from build123d import *

# Parameters (mm, degrees)
BOSS_EXTRUDE1_DEPTH   = 10
FILLET1_R             = 2
F_3_0MM_DOWEL_HOLE1_D = 3.5
F_3_0MM_DOWEL_HOLE2_D = 3.5


with BuildPart() as part:
    # Sketch1 → Boss-Extrude1 (new body)
    with BuildSketch(Plane.XY):
        Polygon((0, 0), (14, 0), (14, 42), (25, 42), (25, 45), (11, 45), (11, 3), (0, 3), align=None)
    extrude(amount=-BOSS_EXTRUDE1_DEPTH)

    # Fillet1
    fillet1_edges = [part.edges().sort_by_distance(p)[0] for p in [
        (11, 3, -5),
        (11, 45, -5),
        (14, 42, -5),
        (14, 0, -5),
    ]]
    fillet(fillet1_edges, radius=FILLET1_R)

    # Ø3.0mm Dowel Hole1 (through all)
    with Locations(Plane(origin=(4.5, 0, -5), x_dir=(0, 0, -1), z_dir=(0, -1, 0))):
        with Locations((0, 0)):
            Hole(F_3_0MM_DOWEL_HOLE1_D / 2)

    # Ø3.0mm Dowel Hole2 (through all)
    with Locations(Plane(origin=(0, 45, 0), x_dir=(1, 0, 0), z_dir=(0, 1, 0))):
        with Locations((20.5, 5)):
            Hole(F_3_0MM_DOWEL_HOLE2_D / 2)


solid = part.part
The listing builds one solid part. Answer for the finished solid, in the listing's coordinates (mm). A direction names the side the tool comes from. Coordinates: 2 decimals unless noted, no trailing zeros. Loops run counter-clockwise (first coordinate to the right, second up) from the corner with the lowest first, then second, coordinate; pieces in that order, holes last. Notation, with made-up numbers: (61, 65.5) -> (78, 65.5) arc R24 cw to (78, 79.5) -> close; hole circle Ø7 at (77, -38). An arc over 180 degrees is marked (long way). Write item = value, one per line. Start each with the question number.
1) A cutting plane is placed at A-A (z = -5). Give the vertices of the cut face in (x, y), then the cut area to 3 significant figures.
2) The mould has two halves that part along X. Classify faces 4 (the face through (10.43, 3.6, -5.07)), 5 (the face through (21.89, 43.48, -3.94)), 6 (the face through (12, 23, -10)): released by +X, released by -X, zero draft, split by the parting line, or undercut.
3) A cutting plane is placed at C-C (z = -2.5). Give the vertices of the cut face in (x, y), then the cut area to 3 significant figures.
4) Straight lines are drawn through the part: line 1 (X direction, y = 42.8, z = -5); line 2 (Y direction, x = 2, z = -7); line 3 (X direction, y = 22.5, z = -6.75). For each, find the intervals that lie inside material, in ascending order. Write a range as from..to.
5) Given pin 1 Ø1.5 at (y, z) = (29, -4) entering from +X; pin 2 Ø5 at (x, z) = (17, -8) entering from -Y; pin 3 Ø1.5 at (y, z) = (40, -5) entering from +X, each flat-ended and moving along its own axis, determine where each tip first touches the part or whether it passes through.
6) A tool of negligible diameter and unlimited length cuts with its end or side. For faces 1 (the face through (0, 2, -5)), 2 (the face through (18, 42, -5)), 3 (the face through (11, 24, -5)), from which of +Z, -Z, +X, -X, +Y, -Y can it reach the whole face along a straight path? Write none if from no direction.
7) A cutting plane is placed at B-B (x = 20.5). Give the vertices of the cut face in (y, z), then the cut area to 3 significant figures.
8) A cutting plane is placed at D-D (y = 23). Give the vertices of the cut face in (x, z), then the cut area to 3 significant figures.
Responses:
q1.outline = (0, 0) -> (2.75, 0) -> (2.75, 3) -> (0, 3) -> close; (6.25, 0) -> (12, 0) arc R2 ccw to (14, 2) -> (14, 40) arc R2 cw to (16, 42) -> (18.75, 42) -> (18.75, 45) -> (13, 45) arc R2 ccw to (11, 43) -> (11, 5) arc R2 cw to (9, 3) -> (6.25, 3) -> close; (22.25, 42) -> (25, 42) -> (25, 45) -> (22.25, 45) -> close
q1.area = 180 mm²
q2.face_4 = released by -X
q2.face_5 = undercut
q2.face_6 = zero draft
q3.outline = (0, 0) -> (12, 0) arc R2 ccw to (14, 2) -> (14, 40) arc R2 cw to (16, 42) -> (25, 42) -> (25, 45) -> (13, 45) arc R2 ccw to (11, 43) -> (11, 5) arc R2 cw to (9, 3) -> (0, 3) -> close
q3.area = 201 mm²
q4.line_1 = 11..18.75, 22.25..25
q4.line_2 = 0..3
q4.line_3 = 11..14
q5.pin_1 = 14
q5.pin_2 = 41.32
q5.pin_3 = 14.15
q6.face_1 = +Z, -Z, -X, +Y, -Y
q6.face_2 = +Z, -Z, +X, -Y
q6.face_3 = +Z, -Z, -X, +Y
q7.outline = (42, -10) -> (45, -10) -> (45, -6.75) -> (42, -6.75) -> close; (42, -3.25) -> (45, -3.25) -> (45, 0) -> (42, 0) -> close
q7.area = 19.5 mm²
q8.outline = (11, -10) -> (14, -10) -> (14, 0) -> (11, 0) -> close
q8.area = 30.0 mm²
